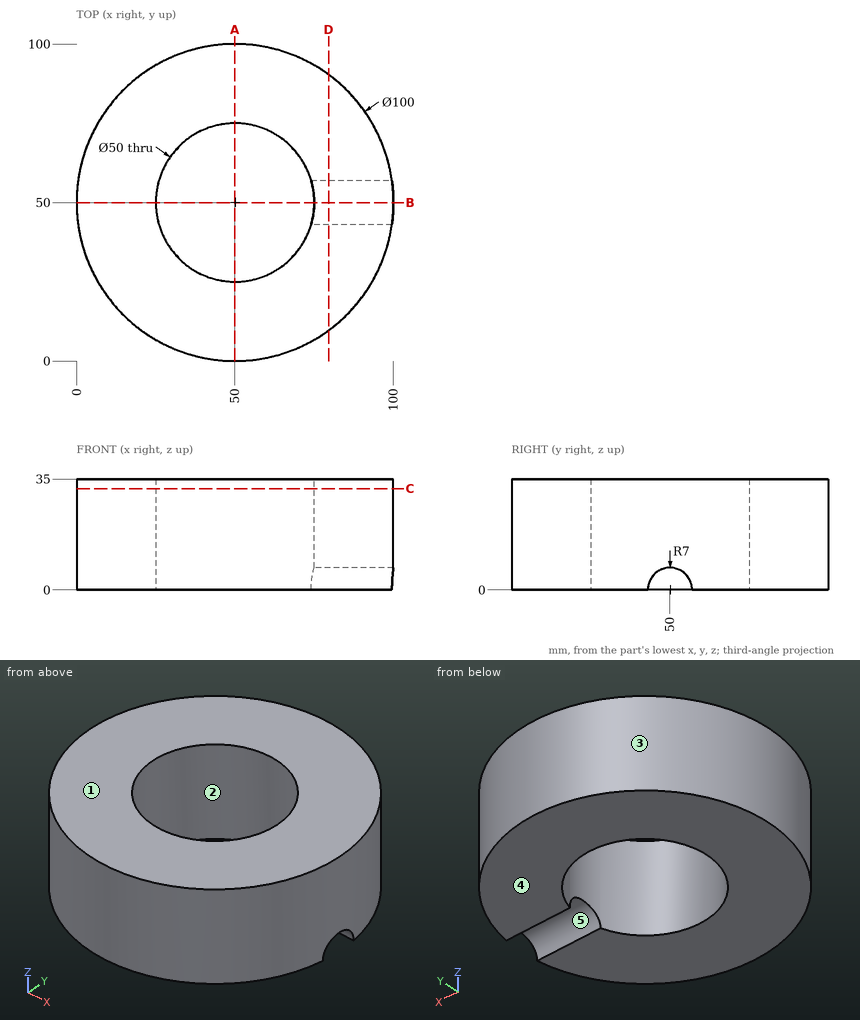
Print and shaded views of the part. All mm, measured from the part's lowest x, y and z. A direction names the side the tool comes from. Coordinates: 2 decimals unless noted, no trailing zeros. Loops run counter-clockwise (first coordinate to the right, second up) from the corner with the lowest first, then second, coordinate; pieces in that order, holes last. Notation, with made-up numbers: (-38.5, 41.25) - (19.5, 41.25) arc R30 cw to (19.5, 77.25) - close; hole circle Ø7 at (60.5, 78). An arc over 180 degrees is marked (long way). Write item = value, one per line. Start each with the question number.
Item 1: Cut at C-C, the plane z = 32. Give the cut face in (x, y).
Item 2: 3-axis set-ups, long thin cutter, end or side, ignore diameter. For the marked faces 4 and 5: which of +Z, -Z, +X, -X, +Y, -Y reach the whole face in a straight line?
Item 3: Cut at A-A, the plane x = 50. Give the cut face in (y, z), and give its area (3 significant figures).
Item 4: Cut at B-B, the plane y = 50. Give the cut face in (x, z).
Item 5: Flat gauge pins, fed straight in: pin 1 Ø2 at (y, z) = (31, 20) entering from -X; pin 2 Ø5 at (y, z) = (86, 8) entering from -X; pin 3 Ø12 at (y, z) = (22.5, 19.5) entering from +X. Where does each tip first touch, or does it go through?
Item 6: Cut at D-D, the plane x = 79.5. Give the cut face in (y, z), and give its area (3 significant figures).
Item 7: Mould opens along X. For the marked faces 1, 2 and 3 say: released by +X, released by -X, zero draft, split by the parting line, or undercut.
Item 8: Wall check: L1, parallel to Y at x = 50, z = 25; L2, parallel to Y at x = 31, z = 18; L3, parallel to X at y = 56.5, z = 12. Give the ranges that are in metal, low to high. Write a range as from..to.
The answers:
q1.outline = circle Ø100 at (50, 50); hole circle Ø50 at (50, 50)
q2.face_4 = -Z, +X, -X, +Y, -Y
q2.face_5 = -Z, +X
q3.outline = (0, 0) - (25, 0) - (25, 35) - (0, 35) - close; (75, 0) - (100, 0) - (100, 35) - (75, 35) - close
q3.area = 1,750 mm2
q4.outline = (0, 0) - (25, 0) - (25, 35) - (0, 35) - close; (75, 7) - (100, 7) - (100, 35) - (75, 35) - close
q5.pin_1 = 3.35
q5.pin_2 = 12.88
q5.pin_3 = 95.14
q6.outline = (9.63, 0) - (43, 0) arc R7 cw to (57, 0) - (90.37, 0) - (90.37, 35) - (9.63, 35) - close
q6.area = 2,750 mm2
q7.face_1 = zero draft
q7.face_2 = undercut
q7.face_3 = split by the parting line
q8.L1 = 0..25, 75..100
q8.L2 = 3.75..33.75, 66.25..96.25
q8.L3 = 0.42..25.86, 74.14..99.58
